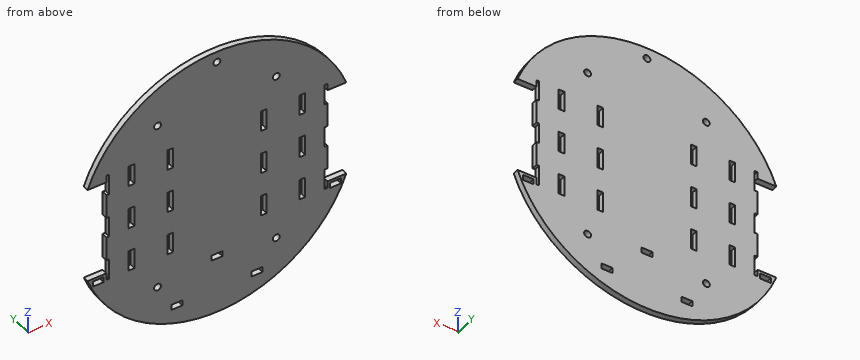
from build123d import *

# Parameters (mm, degrees)
BASE_DEPTH                = 5.334
SKETCH9_W                 = 10
SKETCH9_H                 = 5
TAPE_SENSOR_CUTOUTS_DEPTH = 175.099537782
SKETCH6_W                 = 5.334
SKETCH6_H                 = 19.05
SKETCH6_W_2               = 2.4638
RIGHT_MOUNT_SLOTS_DEPTH   = 175.099537782
SKETCH7_W                 = 5.334
SKETCH7_H                 = 19.05
SKETCH7_W_2               = 2.4638
LEFT_MOUNT_SLOTS_DEPTH    = 175.099537782
SKETCH8_R                 = 3.175
CASTER_SCREWS_DEPTH       = 175.099537782
HOLE1_OUTLINE_R           = 3.175
HOLE1_DEPTH               = 5.334


# Read off the part's stored shape, not the designer's step: Hole1
with BuildPart() as part:
    # Sketch1 → Base (new body)
    with BuildSketch(Plane(origin=(0, 0, 0), x_dir=(1, 0, 0), z_dir=(0, 1, 0))):
        with BuildLine():
            Line((118.967211869, -44.45), (101.6, -44.45))
            Line((101.6, -44.45), (101.6, 44.45))
            Line((101.6, 44.45), (118.967211869, 44.45))
            ThreePointArc((118.967211869, 44.45), (0, 127), (-118.967211869, 44.45))
            Line((-118.967211869, 44.45), (-101.6, 44.45))
            Line((-101.6, 44.45), (-101.6, -44.45))
            Line((-101.6, -44.45), (-118.967211869, -44.45))
            ThreePointArc((-118.967211869, -44.45), (0, -127), (118.967211869, -44.45))
        make_face()
    extrude(amount=BASE_DEPTH)

    # Sketch9 → Tape Sensor Cutouts (cut, through all)
    with BuildSketch(Plane(origin=(0, 5.334, 0), x_dir=(1, 0, 0), z_dir=(0, 1, 0))):
        with Locations((-36.75, 104.1)):
            Rectangle(SKETCH9_W, SKETCH9_H)
        with Locations((36.75, 104.1)):
            Rectangle(SKETCH9_W, SKETCH9_H)
        with Locations((0, 72.35)):
            Rectangle(SKETCH9_W, SKETCH9_H)
        with Locations((-109.14, 49.49)):
            Rectangle(SKETCH9_W, SKETCH9_H)
        with Locations((109.14, 49.49)):
            Rectangle(SKETCH9_W, SKETCH9_H)
    extrude(amount=-TAPE_SENSOR_CUTOUTS_DEPTH, mode=Mode.SUBTRACT)

    # Sketch6 → Right Mount Slots (cut, through all)
    with BuildSketch(Plane.XZ):
        with Locations((42.967, 41.275)):
            Rectangle(SKETCH6_W, SKETCH6_H)
        with Locations((42.967, 0)):
            Rectangle(SKETCH6_W, SKETCH6_H)
        with Locations((42.967, -41.275)):
            Rectangle(SKETCH6_W, SKETCH6_H)
        with Locations((100.3681, 41.275)):
            Rectangle(SKETCH6_W_2, SKETCH6_H)
        with Locations((100.3681, 0)):
            Rectangle(SKETCH6_W_2, SKETCH6_H)
        with Locations((100.3681, -41.275)):
            Rectangle(SKETCH6_W_2, SKETCH6_H)
        with Locations((78.4692, 41.275)):
            Rectangle(SKETCH6_W, SKETCH6_H)
        with Locations((78.4692, 0)):
            Rectangle(SKETCH6_W, SKETCH6_H)
        with Locations((78.4692, -41.275)):
            Rectangle(SKETCH6_W, SKETCH6_H)
    extrude(amount=-RIGHT_MOUNT_SLOTS_DEPTH, mode=Mode.SUBTRACT)

    # Sketch7 → Left Mount Slots (cut, through all)
    with BuildSketch(Plane.XZ):
        with Locations((-78.4692, 0)):
            Rectangle(SKETCH7_W, SKETCH7_H)
        with Locations((-78.4692, 41.275)):
            Rectangle(SKETCH7_W, SKETCH7_H)
        with Locations((-78.4692, -41.275)):
            Rectangle(SKETCH7_W, SKETCH7_H)
        with Locations((-42.967, 41.275)):
            Rectangle(SKETCH7_W, SKETCH7_H)
        with Locations((-42.967, 0)):
            Rectangle(SKETCH7_W, SKETCH7_H)
        with Locations((-42.967, -41.275)):
            Rectangle(SKETCH7_W, SKETCH7_H)
        with Locations((-100.3681, 41.275)):
            Rectangle(SKETCH7_W_2, SKETCH7_H)
        with Locations((-100.3681, 0)):
            Rectangle(SKETCH7_W_2, SKETCH7_H)
        with Locations((-100.3681, -41.275)):
            Rectangle(SKETCH7_W_2, SKETCH7_H)
    extrude(amount=-LEFT_MOUNT_SLOTS_DEPTH, mode=Mode.SUBTRACT)

    # Sketch8 → Caster Screws (cut, through all)
    with BuildSketch(Plane(origin=(0, 5.334, 0), x_dir=(1, 0, 0), z_dir=(0, 1, 0))):
        with Locations(Location((0, -116.84, 0), (0, 0, 270))):
            Circle(SKETCH8_R)
    extrude(amount=-CASTER_SCREWS_DEPTH, mode=Mode.SUBTRACT)

    # Hole1 outline → Hole1 (cut)
    with BuildSketch(Plane(origin=(0, 0, 0), x_dir=(1, 0, 0), z_dir=(0, 1, 0))):
        with Locations((-54.61, -78.74)):
            Circle(HOLE1_OUTLINE_R)
        with Locations((54.61, -78.74)):
            Circle(HOLE1_OUTLINE_R)
        with Locations((54.61, 78.74)):
            Circle(HOLE1_OUTLINE_R)
        with Locations((-54.61, 78.74)):
            Circle(HOLE1_OUTLINE_R)
    extrude(amount=HOLE1_DEPTH, mode=Mode.SUBTRACT)


solid = part.part
Can you work these out from the model? Positions are in its coordinate system, mm. Give positions to 0.01 mm unless a question says otherwise; leave off trailing zeros. Order: outer loops, then holes, each group sorted by start corner. A loop starts at its lowest first (then second) coordinate and runs counter-clockwise, first axis right, second up. Notation, with made-up numbers: M -14.5,49 L 44.5,49 A22 cw 44.5,77 Z; hole C -17.75,-12.5 d8. An arc over 180 degrees is marked long. One line per question, with ' | ' between items.
Item 1: Suppose I cut it at D-D, the plane y = 1.75. Give the number of separate pieces and of enclosed holes in the cut face, then the cut area to 3 significant figures.
Answer block:
separate pieces: 1 | enclosed holes: 22 | area: 44,700 mm2
Item 2: I'm going to push flat-ended pins straight in: pin 1 Ø2.5 at (y, z) = (3.5, -47.5) entering from -X; pin 2 Ø12 at (x, z) = (76.5, -35.5) entering from -Y; pin 3 Ø2.5 at (x, y) = (-100.5, 3.5) entering from -Z; pin 4 Ø2.5 at (x, y) = (-35, 2.5) entering from -Z. Where does each tip first touch, or does it pass through?
Answer block:
pin 1: stops at x = -118.28 | pin 2: stops at y = 0 | pin 3: stops at z = -79.24 | pin 4: stops at z = -122.43
Item 3: Suppose I cut it at C-C, the plane z = 78.74. Write out the boundary of the cut face in (x, y) (3 decimals).
Answer block:
outline: M -99.644,0 L -57.785,0 L -57.785,5.334 L -99.644,5.334 Z; M -51.435,0 L 51.435,0 L 51.435,5.334 L -51.435,5.334 Z; M 57.785,0 L 99.644,0 L 99.644,5.334 L 57.785,5.334 Z
Item 4: Suppose I cut it at B-B, the plane z = -39.5. Write out the boundary of the cut face in (x, y), then the cut area to 3 significant figures.
Answer block:
outline: M -99.14,0 L -81.14,0 L -81.14,5.33 L -99.14,5.33 Z; M -75.8,0 L -45.63,0 L -45.63,5.33 L -75.8,5.33 Z; M -40.3,0 L 40.3,0 L 40.3,5.33 L -40.3,5.33 Z; M 45.63,0 L 75.8,0 L 75.8,5.33 L 45.63,5.33 Z; M 81.14,0 L 99.14,0 L 99.14,5.33 L 81.14,5.33 Z | area: 944 mm2
Item 5: Suppose I cut it at A-A, the plane x = 0. Write out the boundary of the cut face in (y, z) (3 decimals), then the cut area to 3 significant figures.
Answer block:
outline: M 0,-127 L 5.334,-127 L 5.334,-74.85 L 0,-74.85 Z; M 0,-69.85 L 5.334,-69.85 L 5.334,113.665 L 0,113.665 Z; M 0,120.015 L 5.334,120.015 L 5.334,127 L 0,127 Z | area: 1,290 mm2
Item 6: Please list where these lines run through material, in increasing order: L1, parallel to X at y = 4.4, z = -38.5; L2, parallel to Z at x = 54.61, y = 1.55 (3 decimals); L3, parallel to X at y = 1.85, z = 78.74 (3 decimals).
Answer block:
L1: x = -99.14 to -81.14, -75.8 to -45.63, -40.3 to 40.3, 45.63 to 75.8, 81.14 to 99.14 | L2: z = -114.659 to -81.915, -75.565 to 75.565, 81.915 to 114.659 | L3: x = -99.644 to -57.785, -51.435 to 51.435, 57.785 to 99.644
